Input: part model. Units: mm. Frame: model coordinates. A direction names the side the tool comes from. Give positions to 0.01 mm unless a question says otherwise; leave off trailing zeros. Loops run counter-clockwise (first coordinate to the right, second up) from the corner with the lowest first, then second, coordinate; pieces in that order, holes last. Notation, with made-up numbers: (23, -34.75) - (59, -34.75) arc R26 ccw to (59, -15.75) - close; hole circle Ø10 at (11.25, 2.25). An arc over 180 degrees is marked (long way). Answer as a JSON object with one key per item and string values. Group by question number.
(1) Section query A-A (y = -106). Return loops of the section in (x, z) (3 decimals), plus the area to 3 significant figures.
(2) Mould query, pull axis Y, two halves, no side actions, for faces 1 (the flat face through (-95.25, -89, -9)), 2 (the cylindrical face through (-0.995, 63.492, -9.424)), 3 (the cylindrical face through (-27.715, -21.251, -9.424)). Classes: +Y half, -Y half, draft (parallel to the pull), parting line (faces both ways), or undercut.
(3) Pin query (flat end, axial travel): P1, Ø2, axis at y = 42, z = -5, coming from the +X side; P2, Ø10, axis at y = -18, z = -16, coming from the -X side; P3, Ø5, axis at x = -14, z = -8.5, coming from the +Y side. Return the tip coordinate at first contact, or that it passes through.
(4) Access query for faces 4 (the cylindrical face through (-76.316, -13.373, -0.652)), 5 (the flat face through (-60.325, -100, -9)). Directions: +Z, -Z, +X, -X, +Y, -Y. A direction counts if a zero-diameter tool reaches every point of the face in a straight line with its end or side. Return the directions, or none.
(5) Section query B-B (z = -10.5). Return loops of the section in (x, y) (3 decimals), plus the area to 3 significant figures.
(6) Section query C-C (x = 0). Return loops of the section in (y, z) (3 decimals).
(7) Material intervals for L1, parallel to X at y = -90.5, z = -10.25 (3 decimals); L2, parallel to Y at x = 0, z = -12 (3 decimals); L3, parallel to Y at x = -32, z = -15, sorted ascending.
```python
from build123d import *

# Parameters (mm, degrees)
SKETCH1_R      = 34.925
EXTRUDE1_DEPTH = 19.05
CHAMFER3_SIZE  = 4.7752
FILLET1_R      = 2.286


with BuildPart() as part:
    # Sketch1 → Extrude1 (new body)
    with BuildSketch(Plane.XY):
        with BuildLine():
            Line((-60.325, -74.6252), (-60.325, -125.4252))
            Line((-60.325, -125.4252), (-95.25, -125.4252))
            Line((-95.25, -125.4252), (-95.25, -50.8))
            Line((-95.25, -50.8), (-57.124032384, 27.732560721))
            ThreePointArc((-57.124032384, 27.732560721), (0, 63.5), (57.124032384, 27.732560721))
            Line((57.124032384, 27.732560721), (95.25, -50.8))
            Line((95.25, -50.8), (95.25, -125.4252))
            Line((95.25, -125.4252), (60.325, -125.4252))
            Line((60.325, -125.4252), (60.325, -74.6252))
            ThreePointArc((60.325, -74.6252), (47.625, -61.9252), (34.925, -74.6252))
            Line((34.925, -74.6252), (34.925, -125.4252))
            Line((34.925, -125.4252), (-34.925, -125.4252))
            Line((-34.925, -125.4252), (-34.925, -74.6252))
            ThreePointArc((-34.925, -74.6252), (-47.625, -61.9252), (-60.325, -74.6252))
        make_face()
        Circle(SKETCH1_R, mode=Mode.SUBTRACT)
    extrude(amount=-EXTRUDE1_DEPTH)

    # Chamfer3
    chamfer3_edges = [part.edges().sort_by_distance(p)[0] for p in [
        (0, -125.4252, -19.05),
        (77.7875, -125.4252, -19.05),
        (-77.7875, -125.4252, -19.05),
    ]]
    chamfer(chamfer3_edges, length=CHAMFER3_SIZE)

    # Fillet1
    fillet1_edges = [part.edges().sort_by_distance(p)[0] for p in [
        (-76.187016192, -11.53371964, 0),
        (0, 63.5, 0),
        (76.187016192, -11.53371964, 0),
        (76.187016192, -11.53371964, -19.05),
        (0, 63.5, -19.05),
        (-34.925, 0, -19.05),
        (-34.925, 0, 0),
        (-76.187016192, -11.53371964, -19.05),
    ]]
    fillet(fillet1_edges, radius=FILLET1_R)


solid = part.part
```
Recorded:
{
 "1": {"outline": "(-95.25, -19.05) - (-60.325, -19.05) - (-60.325, 0) - (-95.25, 0) - close; (-34.925, -19.05) - (34.925, -19.05) - (34.925, 0) - (-34.925, 0) - close; (60.325, -19.05) - (95.25, -19.05) - (95.25, 0) - (60.325, 0) - close", "area": "2,660 mm^2"},
 "2": {"face 1": "draft", "face 2": "+Y half", "face 3": "undercut"},
 "3": {"P1": "stops at x = 48.49", "P2": "stops at x = -81.75", "P3": "stops at y = 62.45"},
 "4": {"face 4": "+Z, -X, +Y", "face 5": "+Z, -Z, -Y"},
 "5": {"outline": "(-95.25, -125.425) - (-60.325, -125.425) - (-60.325, -74.625) arc R12.7 cw to (-34.925, -74.625) - (-34.925, -125.425) - (34.925, -125.425) - (34.925, -74.625) arc R12.7 cw to (60.325, -74.625) - (60.325, -125.425) - (95.25, -125.425) - (95.25, -50.8) - (57.124, 27.733) arc R63.5 ccw to (-57.124, 27.733) - (-95.25, -50.8) - close; hole circle Ø69.85 at (0, 0)", "area": "22,200 mm^2"},
 "6": {"outline": "(-125.425, -14.275) - (-120.65, -19.05) - (-37.211, -19.05) arc R2.286 ccw to (-34.925, -16.764) - (-34.925, -2.286) arc R2.286 ccw to (-37.211, 0) - (-125.425, 0) - close; (34.925, -16.764) arc R2.286 ccw to (37.211, -19.05) - (61.214, -19.05) arc R2.286 ccw to (63.5, -16.764) - (63.5, -2.286) arc R2.286 ccw to (61.214, 0) - (37.211, 0) arc R2.286 ccw to (34.925, -2.286) - close"},
 "7": {"L1": "x = -95.25 to -60.325, -34.925 to 34.925, 60.325 to 95.25", "L2": "y = -125.425 to -34.925, 34.925 to 63.5", "L3": "y = -124.7 to -13.99, 13.99 to 54.85"}
}
